Can you work these out from the model? Positions are in its coordinate system, mm. A direction names the side the tool comes from. Give positions to 0.01 mm unless a question says otherwise; leave off trailing zeros. Write each loop counter-clockwise with the first axis right and the second up, starting at its lowest first coordinate (ties: lowest second). Pieces come first, ordered by that corner, then holes. Notation, with made-up numbers: M 84.25,-7.75 L 119.25,-7.75 A13 cw 119.25,-0.75 Z; hole C 19.5,-0.75 d10. An arc over 180 degrees is marked long. Write each question's results on one line, items separated by ' | '.
Autodesk Fusion 360 part; units mm, degrees
sketch "Sketch1" plane through (0, 0, 0) normal (0, 1, 0) x (1, 0, 0)
  circle A0 centre (0, 0) radius 34
  circle A1 centre (0, 0) radius 29
  circle A2 centre (0, 0) radius 22.5
  circle A3 centre (0, 0) radius 5.75
  circle A4 centre (0, 0) radius 2
  circle A5 centre (0, 0) radius 7.5
  line L0 (4.6641, -5.8734) -> (13.4973, -18.002)
  line L1 (3.7575, -6.4909) -> (11.2724, -19.4726)
  line L2 (7.4175, -1.1093) -> (22.2525, -3.3279)
  line L3 (7.5, -0.0155) -> (22.49, -0.6714)
  line L4 (5.492, 5.1076) -> (16.4761, 15.3228)
  line L5 (4.6882, 5.8541) -> (14.5472, 17.1648)
  line L6 (-0.5691, 7.4784) -> (-1.7072, 22.4351)
  line L7 (-1.6538, 7.3154) -> (-4.3499, 22.0755)
  line L8 (-6.2016, 4.2178) -> (-18.6049, 12.6533)
  line L9 (-6.7505, 3.268) -> (-19.9715, 10.363)
  line L10 (-7.1643, -2.2189) -> (-21.4928, -6.6567)
  line L11 (-6.764, -3.2402) -> (-20.5541, -9.1531)
  line L12 (-2.732, -6.9847) -> (-8.1961, -20.9541)
  line L13 (-1.684, -7.3085) -> (-5.6591, -21.7767)
  dimension "d1" = 68
  dimension "d2" = 58
  dimension "d3" = 45
  dimension "d4" = 11.5
  dimension "d5" = 4
  dimension "d6" = 15
  dimension "d8" = 6
  dimension "d10" = 360
extrude "Extrude1" add sketch "Sketch1" along normal blind 17.5 contours A3 makes body 1
extrude "Extrude2" add sketch "Sketch1" along normal mid plane 6 contours A5 bodies 1
extrude "Extrude3" add sketch "Sketch1" along normal mid plane 4 contours A2 A5 L4 L5 | A2 A5 L2 L3 | A2 A5 L6 L7 | A2 A5 L0 L1 | A2 A5 L8 L9 | A2 A5 L12 L13 | A2 A5 L10 L11 bodies 1
extrude "Extrude4" add sketch "Sketch1" along normal mid plane 26.5 separate body contours A0 makes body 2
extrude "Extrude5" add sketch "Sketch1" along normal mid plane 26 contours A1 bodies 1 2
equation "d11 = 3 mm + 14.5 mm"
Item 1: I want a section at C-C, the plane z = -9.5. Please give me the cut outline in (x, y).
Geometry says:
outline: M -32.65,-13.25 L -27.4,-13.25 L -27.4,-13 L -20.4,-13 L -20.4,13 L -27.4,13 L -27.4,13.25 L -32.65,13.25 Z; M -18.36,-2 L -13.97,-2 L -13.97,2 L -18.36,2 Z; M -2.05,-2 L -0.72,-2 L -0.72,2 L -2.05,2 Z; M 7.87,-2 L 10.22,-2 L 10.22,2 L 7.87,2 Z; M 20.4,-13 L 27.4,-13 L 27.4,-13.25 L 32.65,-13.25 L 32.65,13.25 L 27.4,13.25 L 27.4,13 L 20.4,13 Z
Item 2: Thinking about a two-plate mould opening in Z: for faces 4 (the face through (18.28, 0.19, -28.67)), 5 (the face through (25, -13.25, -15)), 6 (the face through (15, -13, 17)), which applies, +Z half, -Z half, draft (parallel to the pull), parting line (faces both ways), or undercut?
Geometry says:
face 4: parting line | face 5: draft | face 6: undercut
Item 3: If I drill on line 1 (X direction, y = 10.5, z = 5); line 2 (X direction, y = -13.05, z = 0); line 3 (Y direction, x = 22, z = 5.5), over which ranges is the centre line in solid material (lowest first)? Write a range as from..to.
Geometry says:
line 1: x = -33.63..-21.94, -2.84..2.84, 21.94..33.63 | line 2: x = -34..-29, 29..34 | line 3: y = -13..13
Item 4: I want a section at B-B, the plane x = 8.5. Please give me the cut outline in (y, z), and give its area (3 significant figures).
Geometry says:
outline: M -13.25,-32.92 L 13.25,-32.92 L 13.25,-27.73 L 13,-27.73 L 13,-20.83 L -13,-20.83 L -13,-27.73 L -13.25,-27.73 Z; M -13.25,27.73 L -13,27.73 L -13,20.83 L 13,20.83 L 13,27.73 L 13.25,27.73 L 13.25,32.92 L -13.25,32.92 Z; M -2,-10.23 L 2,-10.23 L 2,-7.91 L -2,-7.91 Z; M -2,0.06 L 2,0.06 L 2,1.27 L -2,1.27 Z; M -2,11.14 L 2,11.14 L 2,14.68 L -2,14.68 Z | area: 662 mm2
Item 5: I want a section at D-D, the plane y = -1. Give the number of separate pieces and of enclosed holes in the cut face, and give its area (3 significant figures).
Geometry says:
separate pieces: 1 | enclosed holes: 8 | area: 2,310 mm2
Item 6: I want a section at A-A, the plane y = 12. Please give me the cut outline in (x, z), and give its area (3 significant figures).
Geometry says:
outline: C 0,0 d68; C 0,0 d11.5; hole C 0,0 d45; hole C 0,0 d4 | area: 2,130 mm2
Item 7: For faces 1 (the face through (-2, -2, -17)), 2 (the face through (7.46, -0.03, 12.89)), 3 (the face through (-2, 3, 6)), which set-ups out of +Z, -Z, +X, -X, +Y, -Y let a thin tool reach every point of the face, with its end or its side?
Geometry says:
face 1: -Y | face 2: +Y, -Y | face 3: +Y
Item 8: I'm going to push flat-ended pins straight in: pin 1 (1.1 mm diameter, centred on x = -1.5, z = -14.5, fed in from -Y); pin 2 (8 mm diameter, centred on x = 19.5, y = 9, fed in from -Z); pin 3 (2 mm diameter, centred on x = -5, z = 17, fed in from +Y). Where does each tip first touch, or does it pass through?
Geometry says:
pin 1: stops at y = -2 | pin 2: stops at z = -30.26 | pin 3: stops at y = 2
